from build123d import *

# Parameters (mm, degrees)
CROQUIS1_R              = 9.5
SALIENTE_EXTRUIR1_DEPTH = 6


with BuildPart() as part:
    # Croquis1 → Saliente-Extruir1 (new body)
    with BuildSketch(Plane.XY):
        with BuildLine():
            Line((-12.5, 0), (-12.5, -10))
            Line((-12.5, -10), (-7.5, -10))
            Line((-7.5, -10), (-7.5, -15))
            Line((-7.5, -15), (4.5, -15))
            Line((4.5, -15), (4.5, -10))
            Line((4.5, -10), (16.5, -10))
            Line((16.5, -10), (16.5, -15))
            Line((16.5, -15), (28.5, -15))
            Line((28.5, -15), (28.5, -10))
            Line((28.5, -10), (32.978801107, -10))
            Line((32.978801107, -10), (32.978801107, 14.339410909))
            ThreePointArc((32.978801107, 14.339410909), (21.612252248, 26.787916382), (8.184354945, 16.596974545))
            ThreePointArc((8.184354945, 16.596974545), (6.46695714, 13.658442551), (3.266576481, 12.5))
            Line((3.266576481, 12.5), (0, 12.5))
            ThreePointArc((0, 12.5), (-8.838834765, 8.838834765), (-12.5, 0))
        make_face()
        Circle(CROQUIS1_R, mode=Mode.SUBTRACT)
        with Locations((20.478801107, 14.339410909)):
            Circle(CROQUIS1_R, mode=Mode.SUBTRACT)
    extrude(amount=SALIENTE_EXTRUIR1_DEPTH)


solid = part.part
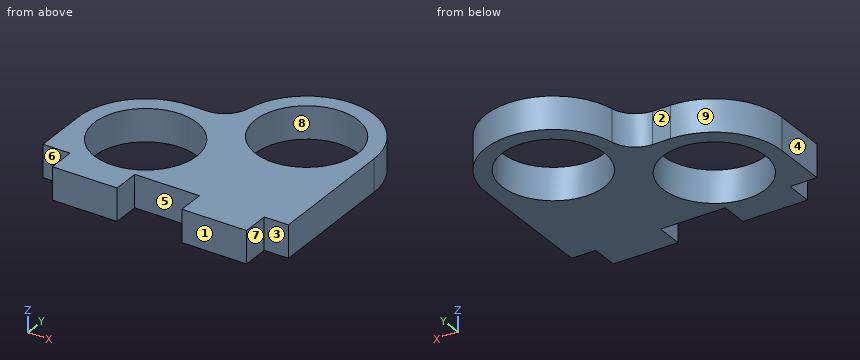
Geometry check sheet. Reference: the model listing, model coordinates, mm. Face numbers are marked on the shaded views. A direction names the side the tool comes from. Give positions to 0.01 mm unless a question says otherwise; leave off trailing zeros. Order: outer loops, then holes, each group sorted by start corner. A loop starts at its lowest first (then second) coordinate and runs counter-clockwise, first axis right, second up. Notation, with made-up numbers: M 39,63.5 L 82,63.5 A24 cw 82,75.5 Z; hole C -27,-3.5 d3. An arc over 180 degrees is marked long. Use a Markdown table: item, result.
Item 1: Draft check along Y on the marked faces 6, 7, 8 and 9. Enter one of: +Y half, -Y half, draft (parallel to the pull), parting line (faces both ways), or undercut.
Answers follow:
| item | result |
|---|---|
| face 6 | -Y half |
| face 7 | draft |
| face 8 | undercut |
| face 9 | +Y half |
Item 2: Material ranges on line 1 along Y through (x, z) = (0, 3.8); line 2 along X through (y, z) = (6, 2.9); line 3 along Y through (x, z) = (20, 0.7), recorded low to high.
Answers follow:
| item | result |
|---|---|
| line 1 | y = -15 to -9.5, 9.5 to 12.5 |
| line 2 | x = -10.97 to -7.37, 7.37 to 15.93, 25.03 to 32.98 |
| line 3 | y = -15 to 4.85, 23.83 to 26.83 |
Item 3: Section check A-A (z = 4.9). Record the cut outline in (x, y).
Answers follow:
| item | result |
|---|---|
| outline | M -12.5,-10 L -7.5,-10 L -7.5,-15 L 4.5,-15 L 4.5,-10 L 16.5,-10 L 16.5,-15 L 28.5,-15 L 28.5,-10 L 32.98,-10 L 32.98,14.34 A12.5 ccw 8.18,16.6 A5 cw 3.27,12.5 L 0,12.5 A12.5 ccw -12.5,0 Z; hole C 0,0 d19; hole C 20.48,14.34 d19 |
Item 4: Section check B-B (y = 19). Record the cut outline in (x, z).
Answers follow:
| item | result |
|---|---|
| outline | M 8.88,0 L 12.2,0 L 12.2,6 L 8.88,6 Z; M 28.76,0 L 32.08,0 L 32.08,6 L 28.76,6 Z |
Item 5: Section check D-D (y = 5.5). Record the cut outline in (x, z), and give its area (3 significant figures).
Answers follow:
| item | result |
|---|---|
| outline | M -11.22,0 L -7.75,0 L -7.75,6 L -11.22,6 Z; M 7.75,0 L 17,0 L 17,6 L 7.75,6 Z; M 23.96,0 L 32.98,0 L 32.98,6 L 23.96,6 Z |
| area | 131 mm2 |
Item 6: Depth check by flat-ended pin: P1, Ø1, axis at x = 2.5, z = 4.5, coming from the +Y side; P2, Ø2, axis at y = 17.5, z = 3, coming from the +X side; P3, Ø1.8, axis at x = 11, z = 2, coming from the -Y side. Enter the tip coordinate at first touch or a pass-through.
Answers follow:
| item | result |
|---|---|
| P1 | stops at y = 12.5 |
| P2 | stops at x = 32.79 |
| P3 | stops at y = -10 |
Item 7: Tool access check on the marked faces 1, 2, 3, 4 and 5. Record the directions out of +Z, -Z, +X, -X, +Y, -Y that give a thin tool (end or side, any length) a straight path to the whole face; none if there is none.
Answers follow:
| item | result |
|---|---|
| face 1 | +Z, -Z, +X, -X, -Y |
| face 2 | +Z, -Z, -X, +Y |
| face 3 | +Z, -Z, +X, -Y |
| face 4 | +Z, -Z, -X, +Y, -Y |
| face 5 | +Z, -Z, -Y |
Item 8: Section check C-C (x = 24.5). Record the cut outline in (y, z), and give its area (3 significant figures).
Answers follow:
| item | result |
|---|---|
| outline | M -15,0 L 5.73,0 L 5.73,6 L -15,6 Z; M 22.95,0 L 26.17,0 L 26.17,6 L 22.95,6 Z |
| area | 144 mm2 |
